Here's how the part is built. I have some questions about the finished solid (model axes, mm). A direction names the side the tool comes from. Round coordinates to 2 decimals unless told otherwise and drop trailing zeros. Order: outer loops, then holes, each group sorted by start corner. A loop starts at its lowest first (then second) coordinate and runs counter-clockwise, first axis right, second up. Notation, with made-up numbers: (29.5, 37) - (40.5, 37) arc R17 ccw to (40.5, 65) - close; hole circle Ø4 at (-29.75, 37). An arc over 180 degrees is marked (long way). Answer as a JSON object with one key per item and string values.
```python
from build123d import *

# Parameters (mm, degrees)
SKETCH1_W           = 210
SKETCH1_H           = 210
SKETCH1_R           = 3
BOSS_EXTRUDE1_DEPTH = 6
SKETCH3_W           = 210
SKETCH3_H           = 6
BOSS_EXTRUDE2_DEPTH = 160
BOSS_EXTRUDE4_DEPTH = 6
BOSS_EXTRUDE5_START = -210
BOSS_EXTRUDE5_DEPTH = 6
SKETCH6_W           = 70
SKETCH6_H           = 100
CUT_EXTRUDE1_DEPTH  = 341.335128954
SKETCH7_W           = 210
SKETCH7_H           = 38
BOSS_EXTRUDE6_DEPTH = 6
SKETCH8_W           = 222
SKETCH8_H           = 206.009708509
BOSS_EXTRUDE7_DEPTH = 6
SKETCH9_W           = 222
SKETCH9_H           = 44
BOSS_EXTRUDE8_DEPTH = 6
CUT_EXTRUDE2_REACH  = 345.965
SKETCH10_R          = 4


with BuildPart() as part:
    # Sketch1 → Boss-Extrude1 (new body)
    with BuildSketch(Plane(origin=(0, 0, 0), x_dir=(1, 0, 0), z_dir=(0, 1, 0))):
        with Locations((105, 105)):
            Rectangle(SKETCH1_W, SKETCH1_H)
        with Locations(Location((62, 179.478184725, 0), (0, 0, 270))):
            Circle(SKETCH1_R, mode=Mode.SUBTRACT)
        with Locations(Location((148, 179.478184725, 0), (0, 0, 270))):
            Circle(SKETCH1_R, mode=Mode.SUBTRACT)
        with Locations(Location((191, 105, 0), (0, 0, 270))):
            Circle(SKETCH1_R, mode=Mode.SUBTRACT)
        with Locations(Location((148, 30.521815275, 0), (0, 0, 270))):
            Circle(SKETCH1_R, mode=Mode.SUBTRACT)
        with Locations(Location((62, 30.521815275, 0), (0, 0, 270))):
            Circle(SKETCH1_R, mode=Mode.SUBTRACT)
        with Locations(Location((19, 105, 0), (0, 0, 270))):
            Circle(SKETCH1_R, mode=Mode.SUBTRACT)
    extrude(amount=BOSS_EXTRUDE1_DEPTH)

    # Sketch3 → Boss-Extrude2 (add)
    with BuildSketch(Plane(origin=(0, 6, 0), x_dir=(1, 0, 0), z_dir=(0, 1, 0))):
        with Locations((105, 3)):
            Rectangle(SKETCH3_W, SKETCH3_H)
    extrude(amount=BOSS_EXTRUDE2_DEPTH)

    # Sketch4 → Boss-Extrude4 (add)
    with BuildSketch(Plane.ZY):
        Polygon((0, 0), (-210, 0), (-210, 44), (-44, 166), (0, 166), align=None)
    extrude(amount=BOSS_EXTRUDE4_DEPTH)

    # Sketch4_3 → Boss-Extrude5 (add)
    with BuildSketch(Plane.ZY.offset(BOSS_EXTRUDE5_START)):
        Polygon((0, 0), (-210, 0), (-210, 44), (-44, 166), (0, 166), align=None)
    extrude(amount=-BOSS_EXTRUDE5_DEPTH)

    # Sketch6 → Cut-Extrude1 (cut, through all)
    with BuildSketch(Plane(origin=(0, 0, -6), x_dir=(-1, 0, 0), z_dir=(0, 0, -1))):
        with Locations((-105, 81)):
            Rectangle(SKETCH6_W, SKETCH6_H)
    extrude(amount=-CUT_EXTRUDE1_DEPTH, mode=Mode.SUBTRACT)

    # Sketch7 → Boss-Extrude6 (add)
    with BuildSketch(Plane(origin=(0, 0, -210), x_dir=(-1, 0, 0), z_dir=(0, 0, -1))):
        with Locations((-105, 25)):
            Rectangle(SKETCH7_W, SKETCH7_H)
    extrude(amount=-BOSS_EXTRUDE6_DEPTH)

    # Sketch8 → Boss-Extrude7 (add)
    with BuildSketch(Plane(origin=(0, 128.779076343, -94.644863336), x_dir=(1, 0, 0), z_dir=(0, 0.8057872670242422, -0.5922050998611905))):
        with Locations((105, 40.153447427)):
            Rectangle(SKETCH8_W, SKETCH8_H)
    extrude(amount=-BOSS_EXTRUDE7_DEPTH)

    # Sketch9 → Boss-Extrude8 (add)
    with BuildSketch(Plane(origin=(0, 166, 0), x_dir=(1, 0, 0), z_dir=(0, 1, 0))):
        with Locations((105, 22)):
            Rectangle(SKETCH9_W, SKETCH9_H)
    extrude(amount=-BOSS_EXTRUDE8_DEPTH)

    # Sketch10 → Cut-Extrude2 (cut, up to next)
    with BuildSketch(Plane.XY, mode=Mode.PRIVATE) as cut_extrude2_sk1:
        with Locations((176, 141)):
            Circle(SKETCH10_R)
    cut_extrude2_tool1 = extrude(cut_extrude2_sk1.sketch, amount=-CUT_EXTRUDE2_REACH, mode=Mode.PRIVATE) & part.part
    # Sketch10 → Cut-Extrude2 (cut, up to next)
    with BuildSketch(Plane.XY, mode=Mode.PRIVATE) as cut_extrude2_sk2:
        with Locations((34, 141)):
            Circle(SKETCH10_R)
    cut_extrude2_tool2 = extrude(cut_extrude2_sk2.sketch, amount=-CUT_EXTRUDE2_REACH, mode=Mode.PRIVATE) & part.part
    # Sketch10 → Cut-Extrude2 (cut, up to next)
    with BuildSketch(Plane.XY, mode=Mode.PRIVATE) as cut_extrude2_sk3:
        with Locations((34, 25)):
            Circle(SKETCH10_R)
    cut_extrude2_tool3 = extrude(cut_extrude2_sk3.sketch, amount=-CUT_EXTRUDE2_REACH, mode=Mode.PRIVATE) & part.part
    # Sketch10 → Cut-Extrude2 (cut, up to next)
    with BuildSketch(Plane.XY, mode=Mode.PRIVATE) as cut_extrude2_sk4:
        with Locations((176, 25)):
            Circle(SKETCH10_R)
    cut_extrude2_tool4 = extrude(cut_extrude2_sk4.sketch, amount=-CUT_EXTRUDE2_REACH, mode=Mode.PRIVATE) & part.part
    add(cut_extrude2_tool1.solids().sort_by_distance((176, 141, 0))[0], mode=Mode.SUBTRACT)
    add(cut_extrude2_tool2.solids().sort_by_distance((34, 141, 0))[0], mode=Mode.SUBTRACT)
    add(cut_extrude2_tool3.solids().sort_by_distance((34, 25, 0))[0], mode=Mode.SUBTRACT)
    add(cut_extrude2_tool4.solids().sort_by_distance((176, 25, 0))[0], mode=Mode.SUBTRACT)


solid = part.part
```
1. Imagine slicing it at A-A (x = 62). List the corners of the cut face in (y, z) for me.
Responses:
{"outline": "(0, -210) - (44, -210) - (166, -44) - (166, 0) - (0, 0) - (0, -27.52) - (6, -27.52) - (6, -6) - (160, -6) - (160, -42.03) - (40.96, -204) - (6, -204) - (6, -182.48) - (0, -182.48) - close; (0, -176.48) - (6, -176.48) - (6, -33.52) - (0, -33.52) - close"}
2. Imagine slicing it at B-B (z = -24.5). List the corners of the cut face in (x, y) for me, plus the area to 3 significant figures.
Responses:
{"outline": "(-6, 0) - (216, 0) - (216, 166) - (-6, 166) - close; hole (0, 6) - (210, 6) - (210, 160) - (0, 160) - close", "area": "4,510 mm2"}
3. Thinking about a two-plate mould opening in Y: for faces 1 (the face through (103, 0, -104)), 2 (the face through (150, 82, -6)), 3 (the face through (0, 67, -82)), 4 (the face through (54, 84, 0)), which applies, pulls with the +Y half, pulls with the -Y half, needs draft (parallel to the pull), parting line crosses it, or undercut?
Responses:
{"face 1": "pulls with the -Y half", "face 2": "undercut", "face 3": "undercut", "face 4": "needs draft"}
4. For P1, Ø3.5, axis at x = 62, z = -30.52, coming from the -Y side; P2, Ø6.5, axis at x = 176, y = 25, coming from the +Z side; P3, Ø12, axis at y = 110.5, z = -137, coming from the +X side; P4, Ø5.5, axis at x = 62, z = -179.48, coming from the -Y side, each with a flat end and sliding along its axis, tell me the tip position at first contact or that it passes through.
Responses:
{"P1": "y = 160", "P2": "z = -204", "P3": "through", "P4": "y = 56.96"}
5. For faces 5 (the face through (105, 31, -3)), 6 (the face through (107, 22, -210)), 7 (the face through (103, 166, -22)), 8 (the face through (62.9, 2.96, -27.66)), 9 (the face through (104, 160, -24)), which set-ups out of +Z, -Z, +X, -X, +Y, -Y let a thin tool reach every point of the face, with its end or its side?
Responses:
{"face 5": "+Z", "face 6": "-Z, +X, -X, +Y, -Y", "face 7": "+Z, -Z, +X, -X, +Y", "face 8": "-Y", "face 9": "none"}
6. If I drill on L1, parallel to Y at x = 176, z = -1; L2, parallel to X at y = 2.7, z = -105; L3, parallel to X at y = 34, z = -51, over which ranges is the centre line in solid material (lowest first)? Write a range as [from, to].
Responses:
{"L1": "[0, 21], [29, 137], [145, 166]", "L2": "[-6, 16], [22, 188], [194, 216]", "L3": "[-6, 0], [210, 216]"}
7. Imagine slicing it at C-C (y = 25). List the corners of the cut face in (x, z) for me, plus the area to 3 significant figures.
Responses:
{"outline": "(-6, -210) - (216, -210) - (216, 0) - (180, 0) - (180, -6) - (210, -6) - (210, -204) - (0, -204) - (0, -6) - (30, -6) - (30, 0) - (-6, 0) - close; (38, -6) - (172, -6) - (172, 0) - (38, 0) - close", "area": "4,940 mm2"}
8. Imagine slicing it at D-D (x = 169). List the corners of the cut face in (y, z) for me, plus the area to 3 significant figures.
Responses:
{"outline": "(0, -210) - (44, -210) - (166, -44) - (166, 0) - (0, 0) - close; hole (6, -204) - (40.96, -204) - (160, -42.03) - (160, -6) - (6, -6) - close", "area": "3,880 mm2"}
